Work out the finished part from the listing and answer in its coordinate system (mm). A direction names the side the tool comes from. Give positions to 0.01 mm unless a question says otherwise; leave off trailing zeros. Loops run counter-clockwise (first coordinate to the right, second up) from the corner with the lowest first, then second, coordinate; pieces in that order, holes last. Notation, with made-up numbers: M 15.25,-26 L 70.25,-26 A13 cw 70.25,-12 Z; hole C -32.75,74.5 d8. An arc over 180 degrees is marked long. Use a Markdown table: item, result.
Solid Edge part; units mm, degrees
sketch "Sketch1" plane through (0, 0, 0) normal (1, 0, 0) x (0, 1, 0)
  line L0 (2.5, 5) -> (2.5, -5)
  line L1 (2.5, -5) -> (10, -5)
  line L2 (10, -5) -> (10, 5)
  line L3 (10, 5) -> (2.5, 5)
  dimension "D1" = 10
revolve "RevolvedProtrusion1" add sketch "Sketch1" angle 360 about axis through (0, 0, -57) along (0, 0, 1)
sketch "Sketch2" plane through (0, 0, 0) normal (0, 0, 1) x (1, 0, 0)
  line L0 (-6, -8) -> (6, -8)
  line L1 (6, -8) -> (10, -35)
  line L2 (10, -35) -> (10, -46)
  line L3 (10, -46) -> (-10, -46)
  line L4 (-10, -46) -> (-10, -35)
  line L5 (-10, -35) -> (-6, -8)
  dimension "D1" = 6
extrude "Protrusion1" add sketch "Sketch2" along normal mid plane 8
sketch "Sketch3" plane through (0, -29, 4) normal (0, 0, 1) x (1, 0, 0)
  line L0 (-10, -17) -> (-10, -6)
  line L1 (-10, -6) -> (10, -6)
  line L2 (10, -6) -> (10, -17)
  line L3 (10, -17) -> (-10, -17)
extrude "ExtrudedProtrusion_2" add sketch "Sketch3" along normal blind 6
hole "Hole_1" at (5, -41.25, -4) direction (0, 0, 1) diameter 4.8 end up to next
hole "Hole1" at (-5, -41.25, -4) direction (0, 0, 1) diameter 4.8 end up to next
sketch "Sketch4" plane through (10, -42.5, 0) normal (1, 0, 0) x (0, 0, -1)
  line L0 (1, -3.5) -> (1, 7.5)
  line L1 (1, 7.5) -> (4, 7.5)
  line L2 (4, 7.5) -> (4, -3.5)
  line L3 (4, -3.5) -> (1, -3.5)
extrude "Cutout1" cut sketch "Sketch4" against normal up to next
chamfer "Chamfer1" distance 3 angle 45 2 edges at (0, -35, -4) (0, -35, 4)
properties material "Polyethylene, low density"
(1) Consider probe 1 along X at (y, z) = (-41.25, 3.25); probe 2 along Z at (x, y) = (-8, -27); probe 3 along X at (y, z) = (-17.5, -2.25). Determine where each line is inside the solid, lowest interval first. Write a range as [from, to].
Entries:
| item | result |
|---|---|
| probe 1 | x = [-10, -7.4], [-2.6, 2.6], [7.4, 10] |
| probe 2 | z = [-4, 4] |
| probe 3 | x = [-7.41, 7.41] |
(2) A cutting plane is placed at C-C (z = 3). Write down the section's boundary in (x, y), and give its area (3 significant figures).
Entries:
| item | result |
|---|---|
| outline | M -10,-46 L 10,-46 L 10,-35 L 6,-8 A10 ccw long -6,-8 L -10,-35 Z; hole C -5,-41.25 d4.8; hole C 0,0 d5; hole C 5,-41.25 d4.8 |
| area | 894 mm² |
(3) The mould has two halves that part along X. Classify faces 6 (the cylindrical face through (-4.894, -43.648, 4.423)), 7 (the flat face through (2, 2, -5)), 8 (the cylindrical face through (-2.44, -0.54, -0.07)), 9 (the flat face through (10, -40, 4)): released by +X, released by -X, zero draft, split by the parting line, or undercut.
Entries:
| item | result |
|---|---|
| face 6 | undercut |
| face 7 | zero draft |
| face 8 | undercut |
| face 9 | released by +X |
(4) A cutting plane is placed at A-A (y = -41.25). Write down the section's boundary in (x, z), and give its area (3 significant figures).
Entries:
| item | result |
|---|---|
| outline | M -10,-1 L -7.4,-1 L -7.4,10 L -10,10 Z; M -2.6,-1 L 2.6,-1 L 2.6,10 L -2.6,10 Z; M 7.4,-1 L 10,-1 L 10,10 L 7.4,10 Z |
| area | 114 mm² |
(5) Given P1, Ø12, axis at x = 2, y = -38.5, coming from the -Z side; P2, Ø6, axis at y = -11.5, z = 2, coming from the -X side; P3, Ø6, axis at x = -6.5, z = -2, coming from the +Y side; P4, Ø4, axis at x = 0, y = 0, coming from the +Z side, each flat-ended and moving along its own axis, determine where each tip first touches the part or whether it passes through.
Entries:
| item | result |
|---|---|
| P1 | stops at z = -3.5 |
| P2 | stops at x = -6.96 |
| P3 | stops at y = 9.37 |
| P4 | passes through |
(6) Which of the six approach directions +Z, -Z, +X, -X, +Y, -Y give full straight-line access (tool end or side, diameter ignored) to faces 1 (the flat face through (0, -41, -1)), 2 (the flat face through (0, -33, 5)), 3 (the flat face through (0, -35, 8)), 4 (the flat face through (7.97, -21.31, 0.2)), 5 (the flat face through (-8.03, -21.69, 0.2))?
Entries:
| item | result |
|---|---|
| face 1 | -Z, +X, -X, -Y |
| face 2 | +Z, +X, -X |
| face 3 | +Z, +X, -X, +Y |
| face 4 | +Z, -Z, +X |
| face 5 | +Z, -Z, -X |
(7) A cutting plane is placed at D-D (y = 0). Write down the section's boundary in (x, z), and give its area (3 significant figures).
Entries:
| item | result |
|---|---|
| outline | M -10,-5 L -2.5,-5 L -2.5,5 L -10,5 Z; M 2.5,-5 L 10,-5 L 10,5 L 2.5,5 Z |
| area | 150 mm² |
